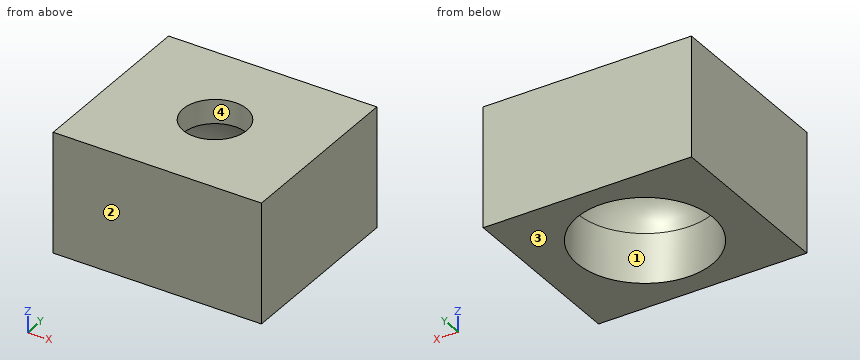
from build123d import *

# Parameters (mm, degrees)
F0_W     = 17.3
F0_H     = 15
F0_R     = 5.65
F1_DEPTH = 10
F2_DEPTH = 8
F3_R     = 2.65
F4_DEPTH = 16.1


# Not quite as in the source:
# - a fillet or chamfer that OpenCascade refuses, or shapes differently, is made with other operations: its cross-section is extruded or revolved along the edge and cut away or added


with BuildPart() as f1:
    # F0 (on Top) → F1 (new body)
    with BuildSketch(Plane.XY):
        Rectangle(F0_W, F0_H)
        Circle(F0_R, mode=Mode.SUBTRACT)
        Circle(F0_R)
    extrude(amount=F1_DEPTH)

    # F0 (on Top) → F2 (cut)
    with BuildSketch(Plane.XY):
        Circle(F0_R)
    extrude(amount=F2_DEPTH, mode=Mode.SUBTRACT)

    # F3 (on face) → F4 (cut)
    with BuildSketch(Plane.XY):
        Circle(F3_R)
    extrude(amount=F4_DEPTH, mode=Mode.SUBTRACT)

    # F5: fillet of radius 4 on 1 edges, made by hand

    # F5_s1 → F5_t2 (revolve)
    with BuildSketch(Plane.XZ):
        with BuildLine():
            ThreePointArc((5.65, 4.1270166538), (4.8122776602, 6.5765063966), (2.65, 8))
            Line((2.65, 8), (5.65, 8))
            Line((5.65, 8), (5.65, 4.1270166538))
        make_face()
    revolve(axis=Axis((0, 0, 8), (0, 0, 1)))


solid = f1.part
Design review of the part built by this model. Coordinates are the model's own, in mm. Face numbers are marked on the shaded views. Give positions to 0.01 mm unless a question says otherwise; leave off trailing zeros. Order: outer loops, then holes, each group sorted by start corner. A loop starts at its lowest first (then second) coordinate and runs counter-clockwise, first axis right, second up.
1. To check wall thickness, follow L1, parallel to X at y = 0, z = 8.6; L2, parallel to Y at x = 0, z = 8.95; L3, parallel to Y at x = 0, z = 3.75. State the ranges of each line that lie inside material, in increasing order.
Solution:
L1: x = -8.65 to -2.65, 2.65 to 8.65
L2: y = -7.5 to -2.65, 2.65 to 7.5
L3: y = -7.5 to -5.65, 5.65 to 7.5
2. Add section A-A, the plane z = 8.5. State the section outline as (x, y) points, then the cut area to 3 significant figures.
Solution:
outline: (-8.65, -7.5) - (8.65, -7.5) - (8.65, 7.5) - (-8.65, 7.5) - close; hole circle Ø5.3 at (0, 0)
area: 237 mm2
3. Mouldability with a two-part tool opening along Y and no side actions: class the marked faces 1, 2, 3 and 4 as +Y half, -Y half, draft (parallel to the pull), parting line (faces both ways), or undercut.
Solution:
face 1: undercut
face 2: -Y half
face 3: draft
face 4: undercut
4. For pin 1 Ø1 at (x, y) = (-2.5, -1) entering from -Z; pin 2 Ø8 at (x, y) = (0.5, 1) entering from -Z, all flat-tipped, find the tip position at first contact; note any pin that passes through.
Solution:
pin 1: stops at z = 7.82
pin 2: stops at z = 6.12
